Can you work these out from the model? Positions are in its coordinate system, mm. Face numbers are marked on the shaded views. A direction names the side the tool comes from. Coordinates: 2 decimals unless noted, no trailing zeros. Order: outer loops, then holes, each group sorted by start corner. A loop starts at its lowest first (then second) coordinate and runs counter-clockwise, first axis right, second up. Notation, with made-up numbers: (49.25, 78) -> (69.25, 78) arc R10 cw to (69.25, 95) -> close; hole circle Ø8 at (56, 36.5). An arc over 180 degrees is marked (long way). Write item = value, one per line.
```python
from build123d import *

# Parameters (mm, degrees)
EXTRUDE_1_DEPTH     = 19.6
SKETCH_2_R          = 3.75
CUT_EXTRUDE_1_DEPTH = 24.783239897


with BuildPart() as part:
    # 草图1 → 凸台-拉伸1 (new body)
    with BuildSketch(Plane(origin=(0, 0, 0), x_dir=(1, 0, 0), z_dir=(0, 1, 0))):
        Polygon((-4.495, 0), (4.495, 0), (9.65, 3.2), (9.65, 6.4), (3.9, 6.4), (3.9, 9.4), (-3.9, 9.4), (-3.9, 6.4), (-9.65, 6.4), (-9.65, 3.2), align=None)
    extrude(amount=EXTRUDE_1_DEPTH)

    # 草图2 → 切除-拉伸1 (cut, through all)
    with BuildSketch(Plane(origin=(0, 0, -9.4), x_dir=(-1, 0, 0), z_dir=(0, 0, -1))):
        with Locations((0, 9.8)):
            Circle(SKETCH_2_R)
    extrude(amount=-CUT_EXTRUDE_1_DEPTH, mode=Mode.SUBTRACT)


solid = part.part
```
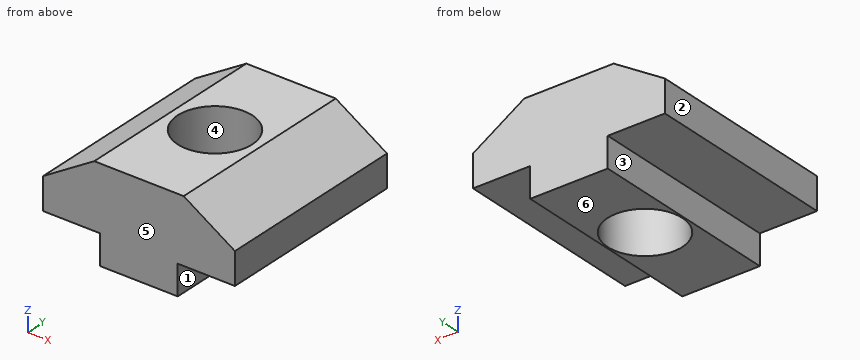
Item 1: I want a section at D-D, the plane y = 17. Please give me the cut outline in (x, z) (3 decimals), plus the area to 3 significant figures.
A:
outline = (-9.65, -6.4) -> (-3.9, -6.4) -> (-3.9, -9.4) -> (3.9, -9.4) -> (3.9, -6.4) -> (9.65, -6.4) -> (9.65, -3.2) -> (4.495, 0) -> (-4.495, 0) -> (-9.65, -3.2) -> close
area = 130 mm2
Item 2: I want a section at A-A, the plane y = 9.8. Please give me the cut outline in (x, z) (3 decimals), plus the area to 3 significant figures.
A:
outline = (-9.65, -6.4) -> (-3.9, -6.4) -> (-3.9, -9.4) -> (-3.75, -9.4) -> (-3.75, 0) -> (-4.495, 0) -> (-9.65, -3.2) -> close; (3.75, -9.4) -> (3.9, -9.4) -> (3.9, -6.4) -> (9.65, -6.4) -> (9.65, -3.2) -> (4.495, 0) -> (3.75, 0) -> close
area = 59.9 mm2
Item 3: I want a section at C-C, the plane z = -5. Please give me the cut outline in (x, y).
A:
outline = (-9.65, 0) -> (9.65, 0) -> (9.65, 19.6) -> (-9.65, 19.6) -> close; hole circle Ø7.5 at (0, 9.8)
Item 4: If I drill on probe 1 along Y at (x, z) = (0, -4.25); probe 2 along X at (y, z) = (13.75, -9); probe 3 along X at (y, z) = (13, -6.5), over which ranges is the centre line in solid material (lowest first)?
A:
probe_1 = 0 to 6.05, 13.55 to 19.6
probe_2 = -3.9 to 3.9
probe_3 = -3.9 to -1.96, 1.96 to 3.9
Item 5: I want a section at B-B, the plane x = 0. Please give me the cut outline in (y, z), plus the area to 3 significant figures.
A:
outline = (0, -9.4) -> (6.05, -9.4) -> (6.05, 0) -> (0, 0) -> close; (13.55, -9.4) -> (19.6, -9.4) -> (19.6, 0) -> (13.55, 0) -> close
area = 114 mm2
Item 6: For the marked faces 1, 2 and 3, which set-ups out of +Z, -Z, +X, -X, +Y, -Y let a thin tool reach every point of the face, with its end or its side?
A:
face_1 = -Z, +X, +Y, -Y
face_2 = +Z, -Z, -X, +Y, -Y
face_3 = -Z, -X, +Y, -Y
Item 7: If we mould it in two halves opening along Y, with no side actions, what happens to the marked faces 4, 5 and 6? For each: pulls with the +Y half, pulls with the -Y half, needs draft (parallel to the pull), parting line crosses it, or undercut.
A:
face_4 = undercut
face_5 = pulls with the -Y half
face_6 = needs draft
Item 8: I'm going to push flat-ended pins straight in: P1, Ø2, axis at y = 15.5, z = -8.5, coming from the -X side; P2, Ø0.9, axis at y = 7, z = -7.5, coming from the +X side. Where does each tip first touch, or does it pass through?
A:
P1 = -3.9
P2 = 3.9
